Verification items for the finished model (mm, model axes). Face numbers are marked on the shaded views. A direction names the side the tool comes from. Coordinates: 2 decimals unless noted, no trailing zeros. Order: outer loops, then holes, each group sorted by start corner. A loop starts at its lowest first (then second) coordinate and runs counter-clockwise, first axis right, second up. Notation, with made-up numbers: (-16, -18) -> (41, -18) arc R15 ccw to (41, -8) -> close; hole circle Ø4 at (60.5, 19.25). An arc over 180 degrees is marked (long way). Write item = value, one per line. Start each with the question number.
from build123d import *

# Parameters (mm, degrees)
F1_DEPTH = 10
F2_W     = 30
F2_H     = 25
F2_W_2   = 20
F2_H_2   = 15
F3_DEPTH = 15
F4_DEPTH = 5


with BuildPart() as f1:
    # F0 (on Top) → F1 (new body)
    with BuildSketch(Plane.XY):
        Polygon((109.8478005826, 31.3216452301), (42.3478005826, 98.8216452301), (42.3478005826, -51.1783547699), (109.8478005826, 16.3216452301), (107.3478005826, 16.3216452301), (107.3478005826, 31.3216452301), align=None)
        Polygon((192.3478005826, 98.8216452301), (42.3478005826, 98.8216452301), (109.8478005826, 31.3216452301), (124.8478005826, 31.3216452301), align=None)
        Polygon((192.3478005826, -51.1783547699), (192.3478005826, 98.8216452301), (124.8478005826, 31.3216452301), (127.3478005826, 31.3216452301), (127.3478005826, 16.3216452301), (124.8478005826, 16.3216452301), align=None)
        Polygon((109.8478005826, 16.3216452301), (42.3478005826, -51.1783547699), (192.3478005826, -51.1783547699), (124.8478005826, 16.3216452301), align=None)
    extrude(amount=F1_DEPTH)

    # F2 (on face) → F3 (join)
    with BuildSketch(Plane.XY.offset(10)):
        with Locations((117.3478005826, 23.8216452301)):
            Rectangle(F2_W, F2_H)
        with Locations((117.3478005826, 23.8216452301)):
            Rectangle(F2_W_2, F2_H_2, mode=Mode.SUBTRACT)
    extrude(amount=F3_DEPTH)

    # F0 (on Top) → F4 (join)
    with BuildSketch(Plane.XY):
        Polygon((127.3478005826, 31.3216452301), (124.8478005826, 31.3216452301), (117.3478005826, 23.8216452301), (124.8478005826, 16.3216452301), (127.3478005826, 16.3216452301), align=None)
        Polygon((124.8478005826, 31.3216452301), (109.8478005826, 31.3216452301), (117.3478005826, 23.8216452301), align=None)
        Polygon((117.3478005826, 23.8216452301), (109.8478005826, 31.3216452301), (107.3478005826, 31.3216452301), (107.3478005826, 16.3216452301), (109.8478005826, 16.3216452301), align=None)
        Polygon((117.3478005826, 23.8216452301), (109.8478005826, 16.3216452301), (124.8478005826, 16.3216452301), align=None)
    extrude(amount=F4_DEPTH)


solid = f1.part
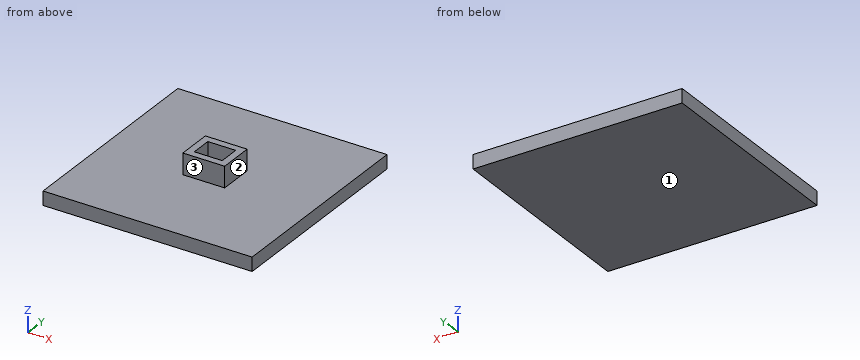
Item 1: Section check C-C (y = -36). Record the boundary of the cut face in (x, z), then the cut area to 3 significant figures.
Item 2: Section check B-B (x = 117). Record the boundary of the cut face in (y, z).
Item 3: Section check A-A (z = 14.75). Record the boundary of the cut face in (x, y).
Item 4: Tool access check on the marked faces 1, 2 and 3. Record the directions out of +Z, -Z, +X, -X, +Y, -Y that give a thin tool (end or side, any length) a straight path to the whole face; none if there is none.
Item 5: Gauge pin test, flat ends, axial feed: P1, Ø6, axis at x = 120.5, z = 18.5, coming from the -Y side; P2, Ø2, axis at x = 67, y = 23.5, coming from the +Z side; P3, Ø7.5, axis at x = 120, y = 21.5, coming from the +Z side. Record the tip position at first contact, or that the pin passes through.
Item 6: Section check D-D (x = 97). Record the boundary of the cut face in (y, z), then the cut area to 3 significant figures.
Item 7: Thickness scan on line 1 (X direction, y = 25, z = 22.75); line 2 (Y direction, x = 107, z = 19.25); line 3 (Z direction, x = 138, y = 9.5). Record the ranges inside material, lowest first.
Filled sheet:
q1.outline = (42.35, 0) -> (192.35, 0) -> (192.35, 10) -> (42.35, 10) -> close
q1.area = 1,500 mm^2
q2.outline = (-51.18, 0) -> (98.82, 0) -> (98.82, 10) -> (36.32, 10) -> (36.32, 25) -> (31.32, 25) -> (31.32, 5) -> (16.32, 5) -> (16.32, 25) -> (11.32, 25) -> (11.32, 10) -> (-51.18, 10) -> close
q3.outline = (102.35, 11.32) -> (132.35, 11.32) -> (132.35, 36.32) -> (102.35, 36.32) -> close; hole (107.35, 16.32) -> (127.35, 16.32) -> (127.35, 31.32) -> (107.35, 31.32) -> close
q4.face_1 = -Z, +X, -X, +Y, -Y
q4.face_2 = +Z, +X, +Y, -Y
q4.face_3 = +Z, +X, -X, -Y
q5.P1 = 11.32
q5.P2 = 10
q5.P3 = 5
q6.outline = (-51.18, 0) -> (98.82, 0) -> (98.82, 10) -> (-51.18, 10) -> close
q6.area = 1,500 mm^2
q7.line_1 = 102.35 to 107.35, 127.35 to 132.35
q7.line_2 = 11.32 to 36.32
q7.line_3 = 0 to 10
